Here's how the part is built. I have some questions about the finished solid (model axes, mm). Give positions to 0.01 mm unless a question says otherwise; leave off trailing zeros. One line per item, written item: value. Start each with the question number.
1) I'm going to push a flat-ended pin straight in: P1, Ø7, axis at x = -651, y = 0, coming from the +Z side. Where does the tip first touch, or does it pass through?
2) Imagine slicing it at A-A on x = -448. Count the separate pieces of the cut face and the enclosed holes in it, plus the area to 3 significant figures.
3) Please list where these lines run through material, in increasing order: L1, parallel to Y at x = 176.5, z = -4.5; L2, parallel to Y at x = -351, z = 11.25; L3, parallel to Z at x = 246, y = 8.25. Write a range as [from, to].
4) We'd pull the mould along Z, two halves only. Please class faces 1 (the flat face through (11, 0, 15)), 2 (the flat face through (11, -6, 0)), 3 (the flat face through (-771, 7, 0)), 4 (the flat face through (11, 6, 0)): +Z half, -Z half, draft (parallel to the pull), parting line (faces both ways), or undercut.
from build123d import *

# Parameters (mm, degrees)
SKETCH_1_W             = 23.5
SKETCH_1_H             = 12
EXTRUDE_1_DEPTH        = 771
HOLE_WIZARD_M6_1_D     = 5
HOLE_WIZARD_M6_1_DEPTH = 15
HOLE_WIZARD_M6_1_TIP   = 1.502151548
HOLE_WIZARD_M6_2_D     = 5
HOLE_WIZARD_M6_2_DEPTH = 15
HOLE_WIZARD_M6_2_TIP   = 1.502151548
SKETCH_7_R             = 4.5
CUT_EXTRUDE_1_DEPTH    = 772.729227126
HOLE_WIZARD_M4_1_D     = 3.3
HOLE_WIZARD_M4_1_DEPTH = 10.1
HOLE_WIZARD_M4_1_TIP   = 0.991420021


with BuildPart() as part:
    # 草图1 → 凸台-拉伸1 (new, symmetric)
    with BuildSketch(Plane(origin=(0, 0, 0), x_dir=(0, 0, -1), z_dir=(1, 0, 0))):
        with BuildLine():
            Line((-14, 15), (-11.5, 15))
            Line((-11.5, 15), (-11.5, 13.5))
            Line((-11.5, 13.5), (-11.4, 13.5))
            ThreePointArc((-11.4, 13.5), (-11.117157288, 13.382842712), (-11, 13.1))
            Line((-11, 13.1), (-11, 12))
            Line((-11, 12), (-9.5, 12))
            Line((-9.5, 12), (-9.5, 15))
            Line((-9.5, 15), (-8, 15))
            Line((-8, 15), (-8, 12.5))
            Line((-8, 12.5), (-5, 12.5))
            Line((-5, 12.5), (-5, 15))
            Line((-5, 15), (5, 15))
            Line((5, 15), (5, 12.5))
            Line((5, 12.5), (8, 12.5))
            Line((8, 12.5), (8, 15))
            Line((8, 15), (9.5, 15))
            Line((9.5, 15), (9.5, 12))
            Line((9.5, 12), (11, 12))
            Line((11, 12), (11, 13.1))
            ThreePointArc((11, 13.1), (11.117157288, 13.382842712), (11.4, 13.5))
            Line((11.4, 13.5), (11.5, 13.5))
            Line((11.5, 13.5), (11.5, 15))
            Line((11.5, 15), (14, 15))
            ThreePointArc((14, 15), (14.707106781, 14.707106781), (15, 14))
            Line((15, 14), (15, 8))
            Line((15, 8), (12.5, 8))
            Line((12.5, 8), (12.5, 5))
            Line((12.5, 5), (15, 5))
            Line((15, 5), (15, -5))
            Line((15, -5), (12.5, -5))
            Line((12.5, -5), (12.5, -8))
            Line((12.5, -8), (15, -8))
            Line((15, -8), (15, -14))
            ThreePointArc((15, -14), (14.707106781, -14.707106781), (14, -15))
            Line((14, -15), (11.5, -15))
            Line((11.5, -15), (11.5, -13.5))
            Line((11.5, -13.5), (11.4, -13.5))
            ThreePointArc((11.4, -13.5), (11.117157288, -13.382842712), (11, -13.1))
            Line((11, -13.1), (11, -12))
            Line((11, -12), (9.5, -12))
            Line((9.5, -12), (9.5, -15))
            Line((9.5, -15), (8, -15))
            Line((8, -15), (8, -12.5))
            Line((8, -12.5), (5, -12.5))
            Line((5, -12.5), (5, -15))
            Line((5, -15), (-5, -15))
            Line((-5, -15), (-5, -12.5))
            Line((-5, -12.5), (-8, -12.5))
            Line((-8, -12.5), (-8, -15))
            Line((-8, -15), (-9.5, -15))
            Line((-9.5, -15), (-9.5, -12))
            Line((-9.5, -12), (-11, -12))
            Line((-11, -12), (-11, -13.1))
            ThreePointArc((-11, -13.1), (-11.117157288, -13.382842712), (-11.4, -13.5))
            Line((-11.4, -13.5), (-11.5, -13.5))
            Line((-11.5, -13.5), (-11.5, -15))
            Line((-11.5, -15), (-14, -15))
            ThreePointArc((-14, -15), (-14.707106781, -14.707106781), (-15, -14))
            Line((-15, -14), (-15, 14))
            ThreePointArc((-15, 14), (-14.707106781, 14.707106781), (-14, 15))
        make_face()
        with BuildLine():
            Line((12, -10.5), (12, -8.5))
            ThreePointArc((12, -8.5), (11.853553391, -8.146446609), (11.5, -8))
            Line((11.5, -8), (-11.5, -8))
            ThreePointArc((-11.5, -8), (-11.853553391, -8.146446609), (-12, -8.5))
            Line((-12, -8.5), (-12, -10.5))
            ThreePointArc((-12, -10.5), (-11.853553391, -10.853553391), (-11.5, -11))
            Line((-11.5, -11), (11.5, -11))
            ThreePointArc((11.5, -11), (11.853553391, -10.853553391), (12, -10.5))
        make_face(mode=Mode.SUBTRACT)
        with BuildLine():
            Line((-11.5, 11), (11.5, 11))
            ThreePointArc((11.5, 11), (11.853553391, 10.853553391), (12, 10.5))
            Line((12, 10.5), (12, 8.5))
            ThreePointArc((12, 8.5), (11.853553391, 8.146446609), (11.5, 8))
            Line((11.5, 8), (-11.5, 8))
            ThreePointArc((-11.5, 8), (-11.853553391, 8.146446609), (-12, 8.5))
            Line((-12, 8.5), (-12, 10.5))
            ThreePointArc((-12, 10.5), (-11.853553391, 10.853553391), (-11.5, 11))
        make_face(mode=Mode.SUBTRACT)
        Rectangle(SKETCH_1_W, SKETCH_1_H, mode=Mode.SUBTRACT)
    extrude(amount=EXTRUDE_1_DEPTH, both=True)

    # M6 螺纹孔1
    with Locations(Plane(origin=(0, 0, -15), x_dir=(-1, 0, 0), z_dir=(0, 0, -1))):
        with Locations((751, 0), (736, 0), (566, 0), (551, 0), (481, 0), (466, 0), (-466, 0), (-481, 0), (-551, 0), (-566, 0), (-736, 0), (-751, 0)):
            Hole(HOLE_WIZARD_M6_1_D / 2, depth=HOLE_WIZARD_M6_1_DEPTH)
            with Locations((0, 0, -(HOLE_WIZARD_M6_1_DEPTH + HOLE_WIZARD_M6_1_TIP / 2))):  # 118° drill point
                Cone(0, HOLE_WIZARD_M6_1_D / 2, HOLE_WIZARD_M6_1_TIP, mode=Mode.SUBTRACT)

    # M6 螺纹孔2
    with Locations(Plane.XZ.offset(15)):
        with Locations((751, 0), (736, 0), (-736, 0), (-751, 0)):
            Hole(HOLE_WIZARD_M6_2_D / 2, depth=HOLE_WIZARD_M6_2_DEPTH)
            with Locations((0, 0, -(HOLE_WIZARD_M6_2_DEPTH + HOLE_WIZARD_M6_2_TIP / 2))):  # 118° drill point
                Cone(0, HOLE_WIZARD_M6_2_D / 2, HOLE_WIZARD_M6_2_TIP, mode=Mode.SUBTRACT)

    # 草图7 → 切除-拉伸1 (cut, through all)
    with BuildSketch(Plane.XY.offset(15)):
        with Locations((-651, 0)):
            Circle(SKETCH_7_R)
        with Locations((-221, 0)):
            Circle(SKETCH_7_R)
        with Locations((651, 0)):
            Circle(SKETCH_7_R)
        with Locations((221, 0)):
            Circle(SKETCH_7_R)
    extrude(amount=-CUT_EXTRUDE_1_DEPTH, mode=Mode.SUBTRACT)

    # M4 螺纹孔1
    with Locations(Plane.XZ.offset(15)):
        with Locations((-151, 0), (-133, 0), (133, 0), (151, 0)):
            Hole(HOLE_WIZARD_M4_1_D / 2, depth=HOLE_WIZARD_M4_1_DEPTH)
            with Locations((0, 0, -(HOLE_WIZARD_M4_1_DEPTH + HOLE_WIZARD_M4_1_TIP / 2))):  # 118° drill point
                Cone(0, HOLE_WIZARD_M4_1_D / 2, HOLE_WIZARD_M4_1_TIP, mode=Mode.SUBTRACT)


solid = part.part
Numbers:
1. P1: through
2. separate pieces: 1
2. enclosed holes: 3
2. area: 407 mm^2
3. L1: [-15, -11], [-8, -6], [6, 8], [11, 15]
3. L2: [-13.47, -11], [-8, -6], [6, 8], [11, 13.47]
3. L3: [-15, -11.93], [11.93, 15]
4. face 1: +Z half
4. face 2: undercut
4. face 3: draft
4. face 4: undercut
